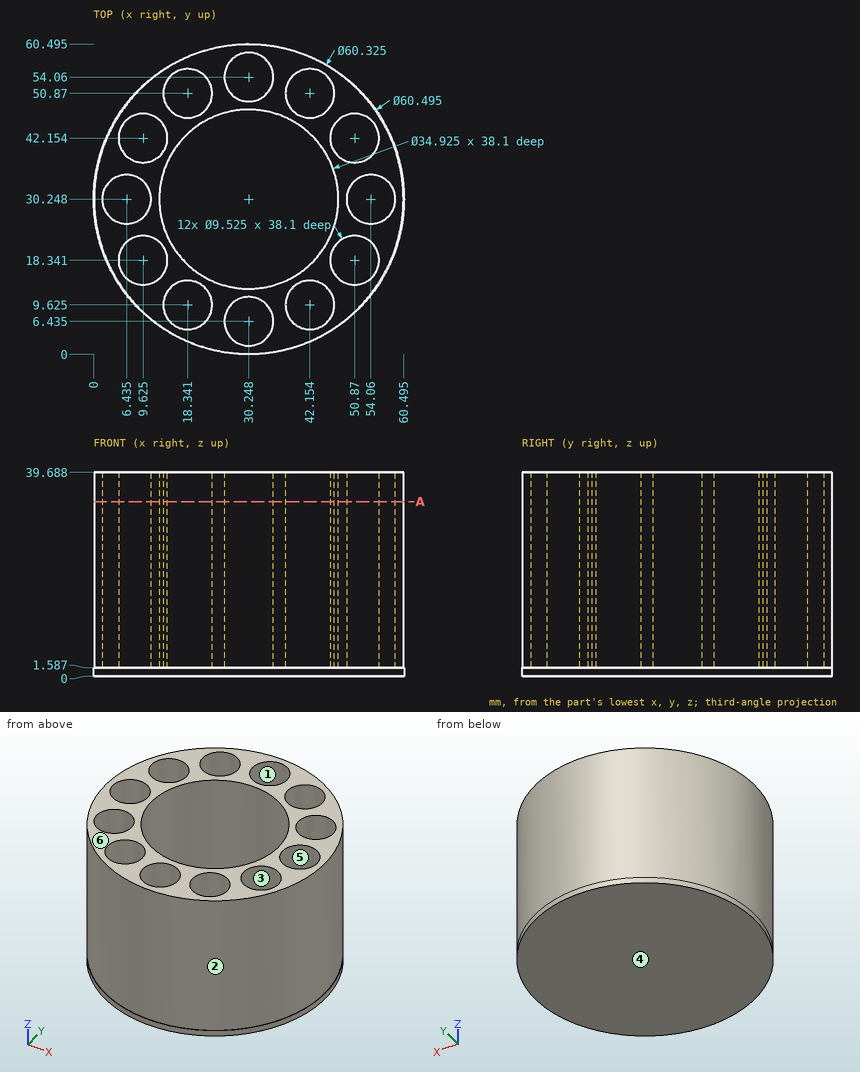
Geometry check sheet. Reference: drawing and pictorial views, mm from the part's lowest x, y, z. A direction names the side the tool comes from. Round coordinates to 2 decimals unless told otherwise and drop trailing zeros.
Item 1: Go/stop test with flat-tipped pins: pin 1 Ø4 at (y, z) = (17.5, 4.5) entering from +X; pin 2 Ø8.5 at (x, y) = (50.87, 18.34) entering from +Z; pin 3 Ø3 at (y, z) = (15.5, 31) entering from +X (1 decimal). Record where each tip stops, or that it passes through.
Determined:
pin 1: stops at x = 58.43
pin 2: stops at z = 1.59
pin 3: stops at x = 57.3
Item 2: Material ranges on line 1 along X through (y, z) = (30, 12) (1 decimal); line 2 along Y through (x, z) = (21, 6) (1 decimal); line 3 along Y through (x, z) = (49, 33) (1 decimal), recorded low to high.
Determined:
line 1: x = 0.1 to 1.7, 11.2 to 12.8, 47.7 to 49.3, 58.8 to 60.4
line 2: y = 1.5 to 5.7, 13.6 to 15.4, 45.1 to 46.9, 54.8 to 59
line 3: y = 6.6 to 14, 22.7 to 37.8, 46.5 to 53.9
Item 3: Access from +Z, -Z, +X, -X, +Y, -Y to the whole of each face (thin tool, end or side, straight path). Record for the marked faces 5 and 6.
Determined:
face 5: +Z
face 6: +Z, +X, -X, +Y, -Y
Item 4: Section check A-A (z = 34). Give the number of separate pieces and of enclosed holes in the cut face.
Determined:
separate pieces: 1
enclosed holes: 13
Item 5: Mould release check, pull along X, two halves, no side actions. Record for the marked faces 1, 2, 3 and 4: +X half, -X half, draft (parallel to the pull), parting line (faces both ways), or undercut.
Determined:
face 1: undercut
face 2: parting line
face 3: undercut
face 4: draft
